Read the model definition and answer for the solid it produces. Units are mm, in the model's axes. Coordinates: 2 decimals unless noted, no trailing zeros. Write each loop counter-clockwise with the first axis right and the second up, starting at its lowest first coordinate (ties: lowest second). Pieces come first, ordered by that corner, then holes.
1) This flat-tipped pin is pushed along its axis until it touches: pin 1 Ø2.5 at (x, y) = (-11.5, 15.5) entering from -Z. Where does it stop, or does it pass through?
2) The part is cut by section B-B (y = 15.5). Determine the outline of the cut face in (x, z).
3) The part is cut by section C-C (z = 0.9). Determine the outline of the cut face in (x, y), then the cut area to 3 significant figures.
4) The part is cut by section A-A (x = -93.5). Determine the outline of the cut face in (y, z), then the cut area to 3 significant figures.
5) Find the intervals of material crossed by line 1 (Y direction, x = -93.5, z = 1.95); line 2 (Y direction, x = -115.09, z = 0.4); line 3 (Y direction, x = -15, z = 2.2), in increasing order.
6) Determine the mould class of faces 1 (the face through (-113.182, 16.101, 0.74)), 2 (the face through (15.496, 15.159, 0.986)), 3 (the face through (-120.496, 15.841, 0.986)) for opening direction X: +X half, -X half, draft (parallel to the pull), parting line (faces both ways), or undercut.
from build123d import *

# Parameters (mm, degrees)
F0_R     = 2
F0_R_2   = 1.5
F1_DEPTH = 3
F2_SIZE  = 1.5
F3_R     = 1


with BuildPart() as f1:
    # F0 (on Top) → F1 (new body)
    with BuildSketch(Plane.XY):
        with BuildLine():
            Line((-105, 0), (0, 0))
            ThreePointArc((0, 0), (15.5, 15.5), (0, 31))
            Line((0, 31), (-105, 31))
            ThreePointArc((-105, 31), (-120.5, 15.5), (-105, 0))
        make_face()
        with Locations((-115.09, 15.5)):
            Circle(F0_R, mode=Mode.SUBTRACT)
        with Locations((-93.5, 15.5)):
            Circle(F0_R_2, mode=Mode.SUBTRACT)
        with Locations((-11.5, 15.5)):
            Circle(F0_R_2, mode=Mode.SUBTRACT)
        with Locations((10.09, 15.5)):
            Circle(F0_R, mode=Mode.SUBTRACT)
    extrude(amount=F1_DEPTH)

    # F2
    f2_edges = [f1.edges().sort_by_distance(p)[0] for p in [
        (-117.09, 15.5, 3),
        (8.09, 15.5, 3),
    ]]
    chamfer(f2_edges, length=F2_SIZE)

    # F3
    f3_edges = [f1.edges().sort_by_distance(p)[0] for p in [
        (-120.5, 15.5, 3),
        (-52.5, 0, 3),
        (-52.5, 31, 3),
        (15.5, 15.5, 3),
    ]]
    fillet(f3_edges, radius=F3_R)


solid = f1.part
Reported:
1. pin 1: passes through
2. outline: (-120.5, 0) - (-117.09, 0) - (-117.09, 1.5) - (-118.59, 3) - (-119.5, 3) arc R1 ccw to (-120.5, 2) - close; (-113.09, 0) - (-95, 0) - (-95, 3) - (-111.59, 3) - (-113.09, 1.5) - close; (-92, 0) - (-13, 0) - (-13, 3) - (-92, 3) - close; (-10, 0) - (8.09, 0) - (8.09, 1.5) - (6.59, 3) - (-10, 3) - close; (12.09, 0) - (15.5, 0) - (15.5, 2) arc R1 ccw to (14.5, 3) - (13.59, 3) - (12.09, 1.5) - close
3. outline: (-105, 0) - (0, 0) arc R15.5 ccw to (0, 31) - (-105, 31) arc R15.5 ccw to start; hole circle Ø4 at (-115.09, 15.5); hole circle Ø3 at (-93.5, 15.5); hole circle Ø3 at (-11.5, 15.5); hole circle Ø4 at (10.09, 15.5)
3. area: 3,970 mm2
4. outline: (0, 0) - (14, 0) - (14, 3) - (1, 3) arc R1 ccw to (0, 2) - close; (17, 0) - (31, 0) - (31, 2) arc R1 ccw to (30, 3) - (17, 3) - close
4. area: 83.6 mm2
5. line 1: y = 0 to 14, 17 to 31
5. line 2: y = 3.73 to 13.5, 17.5 to 27.27
5. line 3: y = 0.02 to 30.98
6. face 1: undercut
6. face 2: +X half
6. face 3: -X half
